from build123d import *

# Parameters (mm, degrees)
SKETCH2_R         = 1.27
EXTRUDE1_DEPTH    = 5.08
CIRPATTERN1_COUNT = 2
SKETCH6_R         = 1.27
EXTRUDE5_DEPTH    = 5.08
EXTRUDE2_REACH    = 66.524
SKETCH4_W         = 7.62
SKETCH4_H         = 3.175
EXTRUDE3_DEPTH    = 0.51
EXTRUDE4_REACH    = 86.92
FILETE1_R         = 1


with BuildPart() as part:
    # Sketch1 → Revolve1 (revolve)
    with BuildSketch(Plane.XY, mode=Mode.PRIVATE) as revolve1_sk:
        Polygon((0, 0), (75, 0), (75, 1.585), (66.3, 1.585), (66.3, 6.5), (61.8, 6.5), (61.8, 17.900000014), (58.5, 17.900000014), (58.5, 19.249999981), (20.5, 19.249999981), (20.5, 17.900000014), (5, 17.900000014), (5, 5.1), (2, 5.1), (2, 1.585), (0, 1.585), align=None)
    revolve(revolve1_sk.sketch.rotate(Axis((0, 0, 0), (1, 0, 0)), 90), axis=Axis((0, 0, 0), (1, 0, 0)))

    # Sketch2 → Extrude1 (cut)
    with BuildSketch(Plane(origin=(61.8, 0, 0), x_dir=(0, 0, -1), z_dir=(1, 0, 0))):
        with Locations((0, 11.84)):
            Circle(SKETCH2_R)
    extrude1 = extrude(amount=-EXTRUDE1_DEPTH, mode=Mode.SUBTRACT)

    # CirPattern1: Extrude1 ×2 about axis
    cirpattern1_axis = Axis((0, 0, 0), (1, 0, 0))
    for i in range(1, CIRPATTERN1_COUNT):
        add(extrude1.rotate(cirpattern1_axis, i * 360 / CIRPATTERN1_COUNT), mode=Mode.SUBTRACT)

    # Sketch6 → Extrude5 (cut)
    with BuildSketch(Plane(origin=(61.8, 0, 0), x_dir=(0, 0, -1), z_dir=(1, 0, 0))):
        with Locations((14.605, 0)):
            Circle(SKETCH6_R)
    extrude(amount=-EXTRUDE5_DEPTH, mode=Mode.SUBTRACT)

    # Sketch3 → Extrude2 (cut, up to next)
    with BuildSketch(Plane(origin=(58.5, 0, 0), x_dir=(0, 0, -1), z_dir=(1, 0, 0)), mode=Mode.PRIVATE) as extrude2_sk1:
        with BuildLine():
            Line((17.863341667, 1.145), (19.863341667, 1.145))
            Line((19.863341667, 1.145), (19.863341667, -1.145))
            Line((19.863341667, -1.145), (17.863341667, -1.145))
            ThreePointArc((17.863341667, -1.145), (17.900000014, 0), (17.863341667, 1.145))
        make_face()
    extrude2_tool1 = extrude(extrude2_sk1.sketch, amount=-EXTRUDE2_REACH, mode=Mode.PRIVATE) & part.part
    add(extrude2_tool1.solids().sort_by_distance((58.5, 0, -18.875533))[0], mode=Mode.SUBTRACT)

    # Sketch4 → Extrude3 (add)
    with BuildSketch(Plane(origin=(0, 15.62, 0), x_dir=(-1, 0, 0), z_dir=(0, 1, 0))):
        with Locations((-1.19, 0)):
            Rectangle(SKETCH4_W, SKETCH4_H)
    extrude3 = extrude(amount=-EXTRUDE3_DEPTH)

    # Sketch5 → Extrude4 (cut, up to next)
    with BuildSketch(Plane(origin=(0, 15.62, 0), x_dir=(1, 0, 0), z_dir=(0, 1, 0)), mode=Mode.PRIVATE) as extrude4_sk1:
        with BuildLine():
            Line((-0.84, 0.635), (1.7, 0.635))
            ThreePointArc((1.7, 0.635), (2.335, 0), (1.7, -0.635))
            Line((1.7, -0.635), (-0.84, -0.635))
            ThreePointArc((-0.84, -0.635), (-1.475, 0), (-0.84, 0.635))
        make_face()
    extrude4_tool1 = extrude(extrude4_sk1.sketch, amount=-EXTRUDE4_REACH, mode=Mode.PRIVATE) & part.part
    extrude4 = extrude4_tool1.solids().sort_by_distance((0.43, 15.62, 0))[0]
    add(extrude4, mode=Mode.SUBTRACT)

    # Mirror1: Extrude3, Extrude4 across plane
    add(extrude3.mirror(Plane.ZX))
    add(extrude4.mirror(Plane.ZX), mode=Mode.SUBTRACT)

    # Filete1
    filete1_edges = [part.edges().sort_by_distance(p)[0] for p in [
        (2, 0, -5.1),
        (61.8, 0, -17.900000014),
        (66.3, 0, -6.5),
    ]]
    fillet(filete1_edges, radius=FILETE1_R)


solid = part.part
Check sheet for the modelled part. Datum: model origin and axes. Units: mm. A direction names the side the tool comes from. Round coordinates to 2 decimals unless told otherwise and drop trailing zeros. Loops run counter-clockwise (first coordinate to the right, second up) from the corner with the lowest first, then second, coordinate; pieces in that order, holes last. Notation, with made-up numbers: (81, 14.25) - (110, 14.25) arc R23 ccw to (110, 30.25) - close; hole circle Ø11 at (51, 61.25). An arc over 180 degrees is marked (long way). Answer as CSV lines item,"result". Start each with the question number.
Item 1: Section check B-B (x = 43). Record the boundary of the cut face in (y, z) (3 decimals).
Item 2: Section check A-A (x = 60). Record the boundary of the cut face in (y, z) (3 decimals).
Item 3: Scan lines: line 1 (Y direction, x = 58.2, z = 0); line 2 (Y direction, x = 59.6, z = 0); line 3 (X direction, y = -10, z = 7.5). Record each from-to range of solid material in increasing order. Write a range as [from, to].
Item 4: Section check C-C (x = 14). Record the boundary of the cut face in (y, z).
Item 5: Release check for a two-part mould opening along Z. For faces 5 (the flat face through (56.72, -12, 0)), 6 (the flat face through (1, -15.62, -1)), 7 (the cylindrical face through (0.99, 1.55, -0.34)) record: +Z half, -Z half, draft (parallel to the pull), parting line (faces both ways), or undercut.
Item 6: Depth check by flat-ended pin: P1, Ø4, axis at y = 2, z = 1.5, coming from the -X side; P2, Ø1.3, axis at y = -12, z = -0.5, coming from the +X side; P3, Ø19, axis at y = -9, z = -8, coming from the -X side; P4, Ø1, axis at x = 1.5, z = -0.5, coming from the -Y side. Enter the tip coordinate at first touch or a pass-through.
Item 7: Set-up check for faces 1 (the cylindrical face through (59.3, -13.1, -0.17)), 2 (the flat face through (1, 15.62, -1)), 3 (the flat face through (20.5, -13, 13)), 4 (the flat face through (1, -15.11, -1)): record each of +Z, -Z, +X, -X, +Y, -Y from which the full face is reachable in a straight line by a thin tool's end or side.
Report:
1,outline,"(-1.145, -19.216) - (-1.145, -17.863) arc R17.9 ccw to (1.145, -17.863) - (1.145, -19.216) arc R19.25 ccw (long way) to start"
2,outline,"circle Ø35.8 at (0, 0); hole circle Ø2.54 at (-11.84, 0); hole circle Ø2.54 at (0, -14.605); hole circle Ø2.54 at (11.84, 0)"
3,line 1,"y = [-19.25, -13.11], [-10.57, 10.57], [13.11, 19.25]"
3,line 2,"y = [-17.9, -13.11], [-10.57, 10.57], [13.11, 17.9]"
3,line 3,"x = [5, 61.8]"
4,outline,"circle Ø35.8 at (0, 0)"
5,face 5,"undercut"
5,face 6,"draft"
5,face 7,"parting line"
6,P1,"stops at x = 0"
6,P2,"stops at x = 56.72"
6,P3,"stops at x = -2.62"
6,P4,"stops at y = -15.62"
7,face 1,"+X"
7,face 2,"+Z, -Z, -X, +Y"
7,face 3,"-X"
7,face 4,"+Z, -Z, -X"
